```python
from build123d import *

# Parameters (mm, degrees)
SKETCH_1_W                         = 50
SKETCH_1_H                         = 70
SM_BASE_FLANGE_1_DEPTH             = 3
SM_EDGE_FLANGE_1_STRIP_W           = 13.4732
SM_EDGE_FLANGE_1_STRIP_H           = 3
SM_EDGE_FLANGE_1_STRIP_CUT_DEPTH   = 50
SM_EDGE_FLANGE_1_STRIP_2_W         = 13.4732
SM_EDGE_FLANGE_1_STRIP_2_H         = 3
SM_EDGE_FLANGE_1_STRIP_CUT_2_DEPTH = 50
SM_EDGE_FLANGE_1_DEPTH             = 50
SM_EDGE_FLANGE_1_BEND_DEPTH        = 50
SM_EDGE_FLANGE_2_STRIP_W           = 13.4732
SM_EDGE_FLANGE_2_STRIP_H           = 3
SM_EDGE_FLANGE_2_STRIP_CUT_DEPTH   = 50
SM_EDGE_FLANGE_2_STRIP_2_W         = 13.4732
SM_EDGE_FLANGE_2_STRIP_2_H         = 3
SM_EDGE_FLANGE_2_STRIP_CUT_2_DEPTH = 50
SM_EDGE_FLANGE_2_DEPTH             = 50
SM_EDGE_FLANGE_2_BEND_DEPTH        = 50
SKETCH_18_R                        = 6.5
CUT_EXTRUDE_1_DEPTH                = 115.144645078


# Sheet-metal steps are written as plain solids
with BuildPart() as part:
    # Sketch 1 → 基体-法兰1 (new body)
    with BuildSketch(Plane.XY):
        with Locations((25, 35)):
            Rectangle(SKETCH_1_W, SKETCH_1_H)
    extrude(amount=-SM_BASE_FLANGE_1_DEPTH)

    # 边线-法兰1 strip (across the edge) → 边线-法兰1 strip cut (cut)
    with BuildSketch(Plane(origin=(0, 70, -3), x_dir=(0, -1, 0), z_dir=(1, 0, 0))):
        with Locations((-6, -1.5)):
            Rectangle(SM_EDGE_FLANGE_1_STRIP_W, SM_EDGE_FLANGE_1_STRIP_H)
    extrude(amount=SM_EDGE_FLANGE_1_STRIP_CUT_DEPTH, mode=Mode.SUBTRACT)

    # 边线-法兰1 strip 2 (across the edge) → 边线-法兰1 strip cut 2 (cut)
    with BuildSketch(Plane(origin=(50, 0, -3), x_dir=(0, 1, 0), z_dir=(-1, 0, 0))):
        with Locations((-6, -1.5)):
            Rectangle(SM_EDGE_FLANGE_1_STRIP_2_W, SM_EDGE_FLANGE_1_STRIP_2_H)
    extrude(amount=SM_EDGE_FLANGE_1_STRIP_CUT_2_DEPTH, mode=Mode.SUBTRACT)

    # 边线-法兰1 section (across the edge) → 边线-法兰1 (add)
    with BuildSketch(Plane(origin=(0, 70, -3), x_dir=(0, -1, 0), z_dir=(1, 0, 0))):
        with BuildLine():
            Line((-3, 0.7366), (-3, 17))
            Line((-3, 17), (0, 17))
            Line((0, 17), (0, 0.7366))
            ThreePointArc((0, 0.7366), (0.215745145, 0.215745145), (0.7366, 0))
            Line((0.7366, 0), (0.7366, -3))
            ThreePointArc((0.7366, -3), (-1.905575199, -1.905575199), (-3, 0.7366))
        make_face()
    extrude(amount=SM_EDGE_FLANGE_1_DEPTH)

    # 边线-法兰1 section 2 (across the edge) → 边线-法兰1 bend (add)
    with BuildSketch(Plane(origin=(50, 0, -3), x_dir=(0, 1, 0), z_dir=(-1, 0, 0))):
        with BuildLine():
            Line((-3, 0.7366), (-3, 17))
            Line((-3, 17), (0, 17))
            Line((0, 17), (0, 0.7366))
            ThreePointArc((0, 0.7366), (0.215745145, 0.215745145), (0.7366, 0))
            Line((0.7366, 0), (0.7366, -3))
            ThreePointArc((0.7366, -3), (-1.905575199, -1.905575199), (-3, 0.7366))
        make_face()
    extrude(amount=SM_EDGE_FLANGE_1_BEND_DEPTH)

    # 边线-法兰2 strip (across the edge) → 边线-法兰2 strip cut (cut)
    with BuildSketch(Plane(origin=(0, -3, -20), x_dir=(0, 0, 1), z_dir=(1, 0, 0))):
        with Locations((-6, -1.5)):
            Rectangle(SM_EDGE_FLANGE_2_STRIP_W, SM_EDGE_FLANGE_2_STRIP_H)
    extrude(amount=SM_EDGE_FLANGE_2_STRIP_CUT_DEPTH, mode=Mode.SUBTRACT)

    # 边线-法兰2 strip 2 (across the edge) → 边线-法兰2 strip cut 2 (cut)
    with BuildSketch(Plane(origin=(50, 73, -20), x_dir=(0, 0, 1), z_dir=(-1, 0, 0))):
        with Locations((-6, -1.5)):
            Rectangle(SM_EDGE_FLANGE_2_STRIP_2_W, SM_EDGE_FLANGE_2_STRIP_2_H)
    extrude(amount=SM_EDGE_FLANGE_2_STRIP_CUT_2_DEPTH, mode=Mode.SUBTRACT)

    # 边线-法兰2 section (across the edge) → 边线-法兰2 (add)
    with BuildSketch(Plane(origin=(0, -3, -20), x_dir=(0, 0, 1), z_dir=(1, 0, 0))):
        with BuildLine():
            Line((-3, 0.7366), (-3, 27))
            Line((-3, 27), (0, 27))
            Line((0, 27), (0, 0.7366))
            ThreePointArc((0, 0.7366), (0.215745145, 0.215745145), (0.7366, 0))
            Line((0.7366, 0), (0.7366, -3))
            ThreePointArc((0.7366, -3), (-1.905575199, -1.905575199), (-3, 0.7366))
        make_face()
    extrude(amount=SM_EDGE_FLANGE_2_DEPTH)

    # 边线-法兰2 section 2 (across the edge) → 边线-法兰2 bend (add)
    with BuildSketch(Plane(origin=(50, 73, -20), x_dir=(0, 0, 1), z_dir=(-1, 0, 0))):
        with BuildLine():
            Line((-3, 0.7366), (-3, 27))
            Line((-3, 27), (0, 27))
            Line((0, 27), (0, 0.7366))
            ThreePointArc((0, 0.7366), (0.215745145, 0.215745145), (0.7366, 0))
            Line((0.7366, 0), (0.7366, -3))
            ThreePointArc((0.7366, -3), (-1.905575199, -1.905575199), (-3, 0.7366))
        make_face()
    extrude(amount=SM_EDGE_FLANGE_2_BEND_DEPTH)

    # 草图18 → 切除-拉伸1 (cut, through all)
    with BuildSketch(Plane.XY):
        with Locations((25, 35)):
            Circle(SKETCH_18_R)
    extrude(amount=-CUT_EXTRUDE_1_DEPTH, mode=Mode.SUBTRACT)


solid = part.part
```
Work out the finished part from the listing and answer in its coordinate system (mm). A direction names the side the tool comes from. Coordinates: 2 decimals unless noted, no trailing zeros. Loops run counter-clockwise (first coordinate to the right, second up) from the corner with the lowest first, then second, coordinate; pieces in that order, holes last.
1) Section B-B (x = 25) is taken. Give the vertices of the cut face in (y, z), plus the area to 3 significant figures.
Results:
outline: (-30, -23) - (-3.74, -23) arc R3.74 ccw to (0, -19.26) - (0, -3.74) arc R0.74 cw to (0.74, -3) - (28.5, -3) - (28.5, 0) - (0.74, 0) arc R3.74 ccw to (-3, -3.74) - (-3, -19.26) arc R0.74 cw to (-3.74, -20) - (-30, -20) - close; (41.5, -3) - (69.26, -3) arc R0.74 cw to (70, -3.74) - (70, -19.26) arc R3.74 ccw to (73.74, -23) - (100, -23) - (100, -20) - (73.74, -20) arc R0.74 cw to (73, -19.26) - (73, -3.74) arc R3.74 ccw to (69.26, 0) - (41.5, 0) - close
area: 459 mm2
2) Section C-C (z = -8.5) is taken. Give the vertices of the cut face in (x, y).
Results:
outline: (0, -3) - (50, -3) - (50, 0) - (0, 0) - close; (0, 70) - (50, 70) - (50, 73) - (0, 73) - close
3) Section A-A (y = 35) is taken. Give the vertices of the cut face in (x, z).
Results:
outline: (0, -3) - (18.5, -3) - (18.5, 0) - (0, 0) - close; (31.5, -3) - (50, -3) - (50, 0) - (31.5, 0) - close
4) Flat-ended cylindrical pins translate along their axes: pin 1 (12.5 mm diameter, centred on x = 18.5, z = -15, fed in from -Y); pin 2 (13 mm diameter, centred on x = 22, y = -18, fed in from +Z); pin 3 (1 mm diameter, centred on x = 12.5, y = -1.5, fed in from +Z); pin 4 (4 mm diameter, centred on x = 42, y = 18.5, fed in from -Z). Find the tip coordinate at first contact, or state that the pin passes through.
Results:
pin 1: stops at y = -30
pin 2: stops at z = -20
pin 3: stops at z = -0.43
pin 4: stops at z = -3
5) For a pull along Y with two mould halves and no side action, classify faces 6 (the flat face through (25, 28, 0)), 7 (the flat face through (25, 0, -12)), 8 (the cylindrical face through (25.35, -1.88, -1.07)) as +Y half, -Y half, draft (parallel to the pull), parting line (faces both ways), or undercut.
Results:
face 6: draft
face 7: undercut
face 8: -Y half
6) Consider probe 1 along Y at (x, z) = (42.5, -16); probe 2 along Y at (x, z) = (25, -2.15); probe 3 along Z at (x, y) = (3, 23). Determine where each line is inside the solid, lowest interval first.
Results:
probe 1: y = -3 to 0, 70 to 73
probe 2: y = -2.65 to 28.5, 41.5 to 72.65
probe 3: z = -3 to 0
7) Section D-D (x = 36) is taken. Give the vertices of the cut face in (y, z).
Results:
outline: (-30, -23) - (-3.74, -23) arc R3.74 ccw to (0, -19.26) - (0, -3.74) arc R0.74 cw to (0.74, -3) - (69.26, -3) arc R0.74 cw to (70, -3.74) - (70, -19.26) arc R3.74 ccw to (73.74, -23) - (100, -23) - (100, -20) - (73.74, -20) arc R0.74 cw to (73, -19.26) - (73, -3.74) arc R3.74 ccw to (69.26, 0) - (0.74, 0) arc R3.74 ccw to (-3, -3.74) - (-3, -19.26) arc R0.74 cw to (-3.74, -20) - (-30, -20) - close
8) For faces 1 (the flat face through (25, 73, -11)), 2 (the flat face through (25, -30, -22)), 3 (the flat face through (25, -3, -11)), 4 (the flat face through (50, 30, -2)), 5 (the flat face through (25, 28, -3)), determine the directions among +Z, -Z, +X, -X, +Y, -Y from which every point of the face is accessible in a straight line to the end or side of a thin tool.
Results:
face 1: +Z, +X, -X, +Y
face 2: +Z, -Z, +X, -X, -Y
face 3: +Z, +X, -X, -Y
face 4: +Z, -Z, +X, +Y, -Y
face 5: -Z, +X, -X
